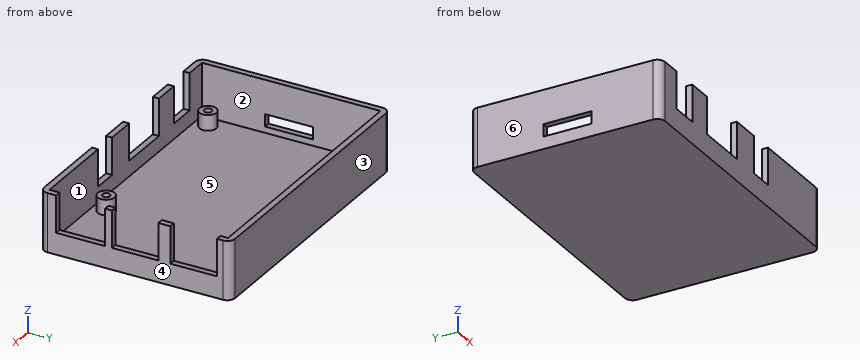
from build123d import *

# Parameters (mm, degrees)
F0_W     = 87
F0_H     = 58
F1_DEPTH = 2
F2_DEPTH = 19
F3_R     = 2.75
F3_R_2   = 1.25
F4_DEPTH = 5
F5_W     = 9
F5_H     = 2
F5_W_2   = 8
F5_W_3   = 17
F5_W_4   = 2
F5_H_2   = 15.9
F5_H_3   = 15.1
F6_DEPTH = 12
F7_W     = 15.6
F7_H     = 4
F8_DEPTH = 2


with BuildPart() as f1:
    # F0 (on Top) → F1 (new body)
    with BuildSketch(Plane.XY):
        with BuildLine():
            ThreePointArc((0, 2.5), (0.732233047, 0.732233047), (2.5, 0))
            Line((2.5, 0), (88.5, 0))
            ThreePointArc((88.5, 0), (90.267766953, 0.732233047), (91, 2.5))
            Line((91, 2.5), (91, 59.5))
            ThreePointArc((91, 59.5), (90.267766953, 61.267766953), (88.5, 62))
            Line((88.5, 62), (2.5, 62))
            ThreePointArc((2.5, 62), (0.732233047, 61.267766953), (0, 59.5))
            Line((0, 59.5), (0, 2.5))
        make_face()
        with Locations((45.5, 31)):
            Rectangle(F0_W, F0_H, mode=Mode.SUBTRACT)
        with Locations((45.5, 31)):
            Rectangle(F0_W, F0_H)
    extrude(amount=F1_DEPTH)

    # F0 (on Top) → F2 (join)
    with BuildSketch(Plane.XY):
        with BuildLine():
            ThreePointArc((0, 2.5), (0.732233047, 0.732233047), (2.5, 0))
            Line((2.5, 0), (88.5, 0))
            ThreePointArc((88.5, 0), (90.267766953, 0.732233047), (91, 2.5))
            Line((91, 2.5), (91, 59.5))
            ThreePointArc((91, 59.5), (90.267766953, 61.267766953), (88.5, 62))
            Line((88.5, 62), (2.5, 62))
            ThreePointArc((2.5, 62), (0.732233047, 61.267766953), (0, 59.5))
            Line((0, 59.5), (0, 2.5))
        make_face()
        with Locations((45.5, 31)):
            Rectangle(F0_W, F0_H, mode=Mode.SUBTRACT)
    extrude(amount=F2_DEPTH)

    # F3 (on face) → F4 (join)
    with BuildSketch(Plane.XY.offset(2)):
        with Locations((6.5, 55.5)):
            Circle(F3_R)
        with Locations((6.5, 55.5)):
            Circle(F3_R_2, mode=Mode.SUBTRACT)
        with Locations((64.5, 55.5)):
            Circle(F3_R)
        with Locations((64.5, 55.5)):
            Circle(F3_R_2, mode=Mode.SUBTRACT)
        with Locations((6.5, 6.5)):
            Circle(F3_R)
        with Locations((6.5, 6.5)):
            Circle(F3_R_2, mode=Mode.SUBTRACT)
        with Locations((64.5, 6.5)):
            Circle(F3_R)
        with Locations((64.5, 6.5)):
            Circle(F3_R_2, mode=Mode.SUBTRACT)
    extrude(amount=F4_DEPTH)

    # F5 (on face) → F6 (cut)
    with BuildSketch(Plane.XY.offset(19)):
        with Locations((13.55, 1)):
            Rectangle(F5_W, F5_H)
        with Locations((57.25, 1)):
            Rectangle(F5_W_2, F5_H)
        with Locations((35, 1)):
            Rectangle(F5_W_3, F5_H)
        with Locations((90, 13.25)):
            Rectangle(F5_W_4, F5_H_2)
        with Locations((90, 30.95)):
            Rectangle(F5_W_4, F5_H_3)
        with Locations((90, 49.95)):
            Rectangle(F5_W_4, F5_H_3)
    extrude(amount=-F6_DEPTH, mode=Mode.SUBTRACT)

    # F7 (on face) → F8 (cut, through all)
    with BuildSketch(Plane(origin=(0, 0, 0), x_dir=(0, -1, 0), z_dir=(-1, 0, 0))):
        with Locations((-30.3, 6)):
            Rectangle(F7_W, F7_H)
    extrude(amount=-F8_DEPTH, mode=Mode.SUBTRACT)


solid = f1.part
The listing builds one solid part. Answer for the finished solid, in the listing's coordinates (mm). Face numbers are marked on the shaded views. A direction names the side the tool comes from. Give positions to 0.01 mm unless a question says otherwise; leave off trailing zeros. Order: outer loops, then holes, each group sorted by start corner. A loop starts at its lowest first (then second) coordinate and runs counter-clockwise, first axis right, second up. Notation, with made-up numbers: (30.5, -23) - (65.5, -23) arc R28 cw to (65.5, 4) - close; hole circle Ø3 at (41, -39.5). An arc over 180 degrees is marked (long way). One line per item, written item: value. Start each with the question number.
1) Find the intervals of material crossed by L1, parallel to Y at x = 6.5, z = 5.25; L2, parallel to Y at x = 82, z = 10.5; L3, parallel to X at y = 40.5, z = 2.25, in increasing order.
2) Given pin 1 Ø1 at (x, z) = (90, 10) entering from -Y; pin 2 Ø10 at (x, y) = (65, 47.5) entering from +Z; pin 3 Ø0.6 at (x, y) = (90, 30.5) entering from +Z, each flat-ended and moving along its own axis, determine where each tip first touches the part or whether it passes through.
3) A cutting plane is placed at D-D on z = 16.75. State how many separate pieces and enclosed holes the cut face has, then the cut area to 3 significant figures.
4) A cutting plane is placed at A-A on x = 36. Give the vertices of the cut face in (y, z).
5) The mould has two halves that part along X. Classify the marked faces 1, 2, 3 and 4: released by +X, released by -X, zero draft, split by the parting line, or undercut.
6) A cutting plane is placed at C-C on x = 6.5. Give the vertices of the cut face in (y, z), then the cut area to 3 significant figures.
7) A cutting plane is placed at B-B on y = 15.5. Give the vertices of the cut face in (x, z), then the cut area to 3 significant figures.
8) A tool of negligible diameter and unlimited length cuts with its end or side. For the marked faces 5 and 6, from which of +Z, -Z, +X, -X, +Y, -Y can it reach the whole face along a straight path? Write none if from no direction.
Answer sheet:
1. L1: y = 0 to 2, 3.75 to 5.25, 7.75 to 9.25, 52.75 to 54.25, 56.75 to 58.25, 60 to 62
1. L2: y = 0 to 2, 60 to 62
1. L3: x = 0 to 2, 89 to 91
2. pin 1: stops at y = 0.21
2. pin 2: stops at z = 2
2. pin 3: stops at z = 7
3. separate pieces: 6
3. enclosed holes: 0
3. area: 430 mm2
4. outline: (0, 0) - (62, 0) - (62, 19) - (60, 19) - (60, 2) - (2, 2) - (2, 7) - (0, 7) - close
5. face 1: undercut
5. face 2: undercut
5. face 3: zero draft
5. face 4: released by +X
6. outline: (0, 0) - (62, 0) - (62, 19) - (60, 19) - (60, 2) - (58.25, 2) - (58.25, 7) - (56.75, 7) - (56.75, 2) - (54.25, 2) - (54.25, 7) - (52.75, 7) - (52.75, 2) - (9.25, 2) - (9.25, 7) - (7.75, 7) - (7.75, 2) - (5.25, 2) - (5.25, 7) - (3.75, 7) - (3.75, 2) - (2, 2) - (2, 19) - (0, 19) - close
6. area: 222 mm2
7. outline: (0, 0) - (91, 0) - (91, 7) - (89, 7) - (89, 2) - (2, 2) - (2, 19) - (0, 19) - close
7. area: 226 mm2
8. face 5: +Z
8. face 6: +Z, -Z, -X, +Y, -Y
